```python
from build123d import *

# Parameters (mm, degrees)
SKETCH1_R           = 40
BOSS_EXTRUDE1_DEPTH = 5
SKETCH2_R           = 1
CUT_EXTRUDE1_DEPTH  = 5
CUT_EXTRUDE2_DEPTH  = 5


with BuildPart() as part:
    # Sketch1 → Boss-Extrude1 (new body)
    with BuildSketch(Plane.XY):
        Circle(SKETCH1_R)
    extrude(amount=BOSS_EXTRUDE1_DEPTH)

    # Sketch2 → Cut-Extrude1 (cut)
    with BuildSketch(Plane.XY):
        with Locations((0, 37)):
            Circle(SKETCH2_R)
        with Locations((0, 22)):
            Circle(SKETCH2_R)
        with Locations((5.694018992, 21.250368178)):
            Circle(SKETCH2_R)
        with Locations((9.576304669, 35.739255573)):
            Circle(SKETCH2_R)
        with Locations((11, 19.052558883)):
            Circle(SKETCH2_R)
        with Locations((18.5, 32.04293994)):
            Circle(SKETCH2_R)
        with Locations((15.556349186, 15.556349186)):
            Circle(SKETCH2_R)
        with Locations((26.162950904, 26.162950904)):
            Circle(SKETCH2_R)
        with Locations((19.052558883, 11)):
            Circle(SKETCH2_R)
        with Locations((32.04293994, 18.5)):
            Circle(SKETCH2_R)
        with Locations((21.250368178, 5.694018992)):
            Circle(SKETCH2_R)
        with Locations((35.739255573, 9.576304669)):
            Circle(SKETCH2_R)
        with Locations((22, 0)):
            Circle(SKETCH2_R)
        with Locations((37, 0)):
            Circle(SKETCH2_R)
        with Locations((21.250368178, -5.694018992)):
            Circle(SKETCH2_R)
        with Locations((35.739255573, -9.576304669)):
            Circle(SKETCH2_R)
        with Locations((19.052558883, -11)):
            Circle(SKETCH2_R)
        with Locations((32.04293994, -18.5)):
            Circle(SKETCH2_R)
        with Locations((15.556349186, -15.556349186)):
            Circle(SKETCH2_R)
        with Locations((26.162950904, -26.162950904)):
            Circle(SKETCH2_R)
        with Locations((11, -19.052558883)):
            Circle(SKETCH2_R)
        with Locations((18.5, -32.04293994)):
            Circle(SKETCH2_R)
        with Locations((5.694018992, -21.250368178)):
            Circle(SKETCH2_R)
        with Locations((9.576304669, -35.739255573)):
            Circle(SKETCH2_R)
        with Locations((0, -22)):
            Circle(SKETCH2_R)
        with Locations((0, -37)):
            Circle(SKETCH2_R)
        with Locations((-5.694018992, -21.250368178)):
            Circle(SKETCH2_R)
        with Locations((-9.576304669, -35.739255573)):
            Circle(SKETCH2_R)
        with Locations((-11, -19.052558883)):
            Circle(SKETCH2_R)
        with Locations((-18.5, -32.04293994)):
            Circle(SKETCH2_R)
        with Locations((-15.556349186, -15.556349186)):
            Circle(SKETCH2_R)
        with Locations((-26.162950904, -26.162950904)):
            Circle(SKETCH2_R)
        with Locations((-19.052558883, -11)):
            Circle(SKETCH2_R)
        with Locations((-32.04293994, -18.5)):
            Circle(SKETCH2_R)
        with Locations((-21.250368178, -5.694018992)):
            Circle(SKETCH2_R)
        with Locations((-35.739255573, -9.576304669)):
            Circle(SKETCH2_R)
        with Locations((-22, 0)):
            Circle(SKETCH2_R)
        with Locations((-37, 0)):
            Circle(SKETCH2_R)
        with Locations((-21.250368178, 5.694018992)):
            Circle(SKETCH2_R)
        with Locations((-35.739255573, 9.576304669)):
            Circle(SKETCH2_R)
        with Locations((-19.052558883, 11)):
            Circle(SKETCH2_R)
        with Locations((-32.04293994, 18.5)):
            Circle(SKETCH2_R)
        with Locations((-15.556349186, 15.556349186)):
            Circle(SKETCH2_R)
        with Locations((-26.162950904, 26.162950904)):
            Circle(SKETCH2_R)
        with Locations((-11, 19.052558883)):
            Circle(SKETCH2_R)
        with Locations((-18.5, 32.04293994)):
            Circle(SKETCH2_R)
        with Locations((-5.694018992, 21.250368178)):
            Circle(SKETCH2_R)
        with Locations((-9.576304669, 35.739255573)):
            Circle(SKETCH2_R)
    extrude(amount=CUT_EXTRUDE1_DEPTH, mode=Mode.SUBTRACT)

    # Sketch5 → Cut-Extrude2 (cut)
    with BuildSketch(Plane.XY):
        with BuildLine():
            Line((-3.25, 2.738612788), (-3.25, -2.738612788))
            ThreePointArc((-3.25, -2.738612788), (0, -4.25), (3.25, -2.738612788))
            Line((3.25, -2.738612788), (3.25, 2.738612788))
            ThreePointArc((3.25, 2.738612788), (0, 4.25), (-3.25, 2.738612788))
        make_face()
    extrude(amount=CUT_EXTRUDE2_DEPTH, mode=Mode.SUBTRACT)


solid = part.part
```
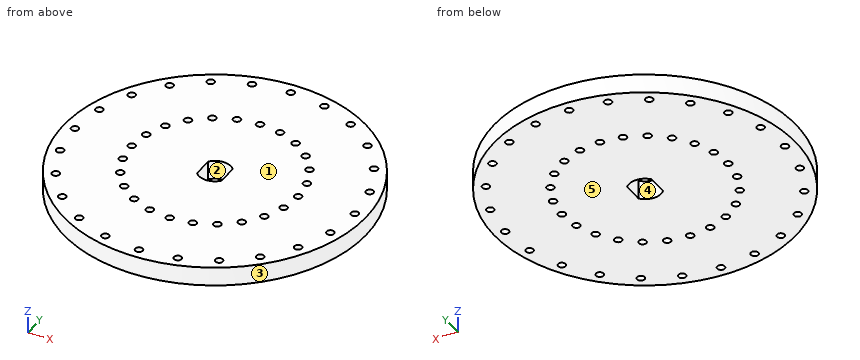
Model file for the job. Use its own axes, mm. Face numbers are marked on the shaded views. A direction names the side the tool comes from. Round coordinates to 2 decimals unless told otherwise and drop trailing zeros. Write each loop counter-clockwise with the first axis right and the second up, starting at its lowest first coordinate (ties: lowest second). Pieces come first, ordered by that corner, then holes. Notation, with made-up numbers: (-17.5, 84.25) -> (37.5, 84.25) arc R19 cw to (37.5, 95.25) -> close; hole circle Ø11 at (81, 27). An arc over 180 degrees is marked (long way). Answer as CSV lines item,"result".
1. Slice it at D-D, the plane y = -28.5. List the corners of the cut face in (x, z), plus the area to 3 significant figures.
Resolved:
outline,"(-28.07, 0) -> (28.07, 0) -> (28.07, 5) -> (-28.07, 5) -> close"
area,"281 mm²"
2. Slice it at A-A, the plane x = 0. List the corners of the cut face in (y, z), plus the area to 4 significant figures.
Resolved:
outline,"(-40, 0) -> (-38, 0) -> (-38, 5) -> (-40, 5) -> close; (-36, 0) -> (-23, 0) -> (-23, 5) -> (-36, 5) -> close; (-21, 0) -> (-4.25, 0) -> (-4.25, 5) -> (-21, 5) -> close; (4.25, 0) -> (21, 0) -> (21, 5) -> (4.25, 5) -> close; (23, 0) -> (36, 0) -> (36, 5) -> (23, 5) -> close; (38, 0) -> (40, 0) -> (40, 5) -> (38, 5) -> close"
area,"317.5 mm²"
3. Slice it at C-C, the plane z = 2.3. State how many separate pieces and enclosed holes the cut face has, plus the area to 3 significant figures.
Resolved:
separate pieces,"1"
enclosed holes,"49"
area,"4,830 mm²"
4. Mould opens along Y. For the marked faces 1, 2 and 3 say: +Y half, -Y half, draft (parallel to the pull), parting line (faces both ways), or undercut.
Resolved:
face 1,"draft"
face 2,"undercut"
face 3,"parting line"
5. Tool access for the marked faces 4 and 5: list every direction of +Z, -Z, +X, -X, +Y, -Y with a clear straight run to the whole face (end or side of a thin tool).
Resolved:
face 4,"+Z, -Z"
face 5,"-Z, +X, -X, +Y, -Y"
6. Pin check, flat tips, straight feed: pin 1 Ø12 at (x, y) = (-22, 16) entering from -Z; pin 2 Ø1 at (x, z) = (20.5, 1.5) entering from -Y. Stop position of each tip, or through.
Resolved:
pin 1,"z = 0"
pin 2,"y = -34.64"
7. Drill centre lines: line 1 (Y direction, x = 0, z = 2.65); line 2 (X direction, y = 36.5, z = 2.5); line 3 (X direction, y = 26, z = 1.9). Where is each one in solid material? Low to high.
Resolved:
line 1,"-40 to -38, -36 to -23, -21 to -4.25, 4.25 to 21, 23 to 36, 38 to 40"
line 2,"-16.36 to -10.23, -8.93 to -0.87, 0.87 to 8.93, 10.23 to 16.36"
line 3,"-30.4 to -27.15, -25.18 to 25.18, 27.15 to 30.4"
8. Slice it at B-B, the plane y = 0. List the corners of the cut face in (x, z).
Resolved:
outline,"(-40, 0) -> (-38, 0) -> (-38, 5) -> (-40, 5) -> close; (-36, 0) -> (-23, 0) -> (-23, 5) -> (-36, 5) -> close; (-21, 0) -> (-3.25, 0) -> (-3.25, 5) -> (-21, 5) -> close; (3.25, 0) -> (21, 0) -> (21, 5) -> (3.25, 5) -> close; (23, 0) -> (36, 0) -> (36, 5) -> (23, 5) -> close; (38, 0) -> (40, 0) -> (40, 5) -> (38, 5) -> close"
